from build123d import *

# Parameters (mm, degrees)
F1_DEPTH    = 25
F2_T1_DEPTH = 37.6241632485
F2_T3_DEPTH = 37.4381172953


# Not quite as in the source:
# - a fillet or chamfer that OpenCascade refuses, or shapes differently, is made with other operations: its cross-section is extruded or revolved along the edge and cut away or added


with BuildPart() as f1:
    # F0 (on Top) → F1 (new body)
    with BuildSketch(Plane.XY):
        with BuildLine():
            ThreePointArc((-150, 0), (0, 50), (150, 0))
            Line((150, 0), (152.7, 3.6))
            ThreePointArc((152.7, 3.6), (0, 54.5), (-152.7, 3.6))
            Line((-152.7, 3.6), (-150, 0))
        make_face()
    extrude(amount=F1_DEPTH)

    # F2: fillet of radius 2.5 on 4 edges, made by hand

    # F2_s2 → F2_t1 (cut)
    with BuildSketch(Plane.XY.offset(-6.3120816242)):
        with BuildLine():
            ThreePointArc((-150.6726442548, 5.1048616519), (-151.6656488685, 3.4559044723), (-151.1925593407, 1.590079121))
            Line((-151.1925593407, 1.590079121), (-152.7, 3.6))
            ThreePointArc((-152.7, 3.6), (-151.6881883097, 4.3549449544), (-150.6726442548, 5.1048616519))
        make_face()
        with BuildLine():
            ThreePointArc((151.1925593407, 1.590079121), (151.6656488685, 3.4559044723), (150.6726442548, 5.1048616519))
            ThreePointArc((150.6726442548, 5.1048616519), (151.6881883097, 4.3549449544), (152.7, 3.6))
            Line((152.7, 3.6), (151.1925593407, 1.590079121))
        make_face()
    extrude(amount=F2_T1_DEPTH, mode=Mode.SUBTRACT)

    # F2_s4 → F2_t3 (cut)
    with BuildSketch(Plane.XY.offset(-6.2190586476)):
        with BuildLine():
            ThreePointArc((-148.0124495796, 1.4753453141), (-149.8583751339, 1.0170056461), (-151.4925740754, 1.9900987672))
            Line((-151.4925740754, 1.9900987672), (-150, 0))
            ThreePointArc((-150, 0), (-149.0080507458, 0.7401325419), (-148.0124495796, 1.4753453141))
        make_face()
        with BuildLine():
            ThreePointArc((148.0124495796, 1.4753453141), (149.8583751339, 1.0170056461), (151.4925740754, 1.9900987672))
            Line((151.4925740754, 1.9900987672), (150, 0))
            ThreePointArc((150, 0), (149.0080507458, 0.7401325419), (148.0124495796, 1.4753453141))
        make_face()
    extrude(amount=F2_T3_DEPTH, mode=Mode.SUBTRACT)


solid = f1.part
Read the model definition and answer for the solid it produces. Units are mm, in the model's axes. Coordinates: 2 decimals unless noted, no trailing zeros. Loops run counter-clockwise (first coordinate to the right, second up) from the corner with the lowest first, then second, coordinate; pieces in that order, holes last. Notation, with made-up numbers: (-33.75, -6) -> (-4.75, -6) arc R15 ccw to (-4.75, 19) -> close; hole circle Ø9 at (-39, 20). An arc over 180 degrees is marked (long way). Answer in a Markdown table with one row per item.
Item 1: A cutting plane is placed at A-A on y = 19. Determine the outline of the cut face in (x, z), plus the area to 3 significant figures.
Returned:
| item | result |
|---|---|
| outline | (-129.65, 0) -> (-120.58, 0) -> (-120.58, 25) -> (-129.65, 25) -> close; (120.58, 0) -> (129.65, 0) -> (129.65, 25) -> (120.58, 25) -> close |
| area | 454 mm^2 |
Item 2: A cutting plane is placed at D-D on x = 33. Determine the outline of the cut face in (y, z).
Returned:
| item | result |
|---|---|
| outline | (47.81, 0) -> (52.35, 0) -> (52.35, 25) -> (47.81, 25) -> close |
Item 3: Straight lines are drawn through the part: line 1 along X through (y, z) = (5, 7.75); line 2 along X through (y, z) = (30.5, 23.75); line 3 along Y through (x, z) = (-81, 10.75). For each, find the intervals that lie inside material, in ascending order. Write a range as [from, to].
Returned:
| item | result |
|---|---|
| line 1 | x = [-150.81, -143.09], [143.09, 150.81] |
| line 2 | x = [-107.89, -96.8], [96.8, 107.89] |
| line 3 | y = [36.51, 41.27] |
Item 4: Each of these flat-tipped pins is pushed along its axis until it touches: P1, Ø1.5, axis at x = -118.5, z = 21.5, coming from the -Y side; P2, Ø6, axis at y = 37, z = 15, coming from the -X side; P3, Ø12, axis at x = -119, z = 6.5, coming from the -Y side. Where does it stop, or does it pass through?
Returned:
| item | result |
|---|---|
| P1 | stops at y = 19.73 |
| P2 | stops at x = -100.07 |
| P3 | stops at y = 16.51 |
Item 5: A cutting plane is placed at B-B on z = 17. Determine the outline of the cut face in (x, y), plus the area to 3 significant figures.
Returned:
| item | result |
|---|---|
| outline | (-151.33, 1.8) arc R2.5 ccw to (-148.01, 1.48) arc R250 cw to (148.01, 1.48) arc R2.5 ccw to (151.33, 1.8) arc R2.5 ccw to (150.67, 5.1) arc R254.5 ccw to (-150.67, 5.1) arc R2.5 ccw to start |
| area | 1,460 mm^2 |
Item 6: A cutting plane is placed at C-C on y = 30. Determine the outline of the cut face in (x, z), plus the area to 3 significant figures.
Returned:
| item | result |
|---|---|
| outline | (-108.95, 0) -> (-97.98, 0) -> (-97.98, 25) -> (-108.95, 25) -> close; (97.98, 0) -> (108.95, 0) -> (108.95, 25) -> (97.98, 25) -> close |
| area | 549 mm^2 |
Item 7: For a pull along X with two mould halves and no side action, classify faces 1 (the cylindrical face through (2.26, 54.49, 12.32)), 2 (the cylindrical face through (-2.22, 49.99, 12.32)), 3 (the flat face through (-1, 52, 0)) as released by +X, released by -X, zero draft, split by the parting line, or undercut.
Returned:
| item | result |
|---|---|
| face 1 | split by the parting line |
| face 2 | undercut |
| face 3 | zero draft |
